Check sheet for the modelled part. Datum: model origin and axes. Units: mm. Coordinates: 2 decimals unless noted, no trailing zeros. Write each loop counter-clockwise with the first axis right and the second up, starting at its lowest first coordinate (ties: lowest second). Pieces come first, ordered by that corner, then holes. Notation, with made-up numbers: M 63.25,14.5 L 122.25,14.5 A9 ccw 122.25,20.5 Z; hole C 0,-29.75 d4. An arc over 180 degrees is marked long. Answer as CSV lines item,"result". Start each with the question number.
Q1. Sectioned sample at B-B, the plane x = 34. Record the cut outline in (y, z).
Q2. Thickness scan on line 1 along Y through (x, z) = (-60.5, -0.85); line 2 along Y through (x, z) = (-5, -0.9); line 3 along Y through (x, z) = (50, 0.05). Record the ranges inside material, lowest first. Write a range as from..to.
Q3. Sectioned sample at A-A, the plane x = 58.9. Record the cut outline in (y, z), then the cut area to 3 significant figures.
Q4. Sectioned sample at C-C, the plane y = 0.05. Record the cut outline in (x, z), then the cut area to 3 significant figures.
Q5. Sectioned sample at D-D, the plane z = -1.45. Count the separate pieces of the cut face and the enclosed holes in it, then the cut area to 3 significant figures.
Q6. Depth check by flat-ended pin: pin 1 Ø3.5 at (x, y) = (-45, 5) entering from +Z. Enter the tip coordinate at first touch or a pass-through.
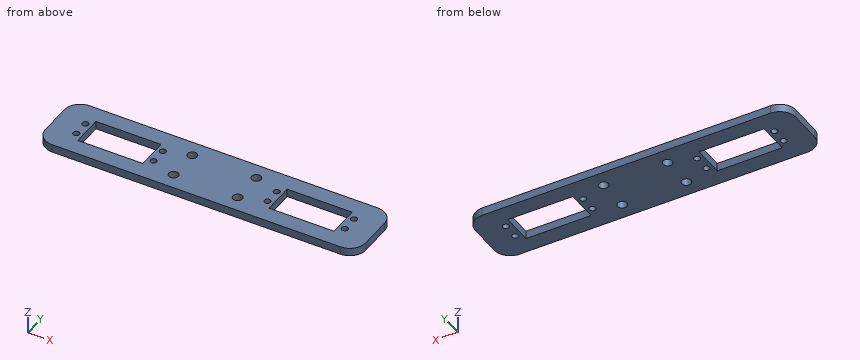
from build123d import *

# Parameters (mm, degrees)
CROQUIS1_W            = 200
CROQUIS1_H            = 40
EXTRUIR1_DEPTH        = 2.5
REDONDEO1_R           = 10
CROQUIS3_W            = 40.6
CROQUIS3_H            = 19.5
EXTRUIR2_DEPTH        = 10
CROQUIS4_R            = 1.95
CORTAR_EXTRUIR1_DEPTH = 10
CROQUIS5_R            = 2.95
CORTAR_EXTRUIR3_DEPTH = 10


with BuildPart() as part:
    # Croquis1 → Extruir1 (new, symmetric)
    with BuildSketch(Plane.XY):
        with Locations((-25, -5)):
            Rectangle(CROQUIS1_W, CROQUIS1_H)
    extrude(amount=EXTRUIR1_DEPTH, both=True)

    # Redondeo1
    redondeo1_edges = [part.edges().sort_by_distance(p)[0] for p in [
        (75, 15, 0),
        (75, -25, 0),
        (-125, -25, 0),
        (-125, 15, 0),
    ]]
    fillet(redondeo1_edges, radius=REDONDEO1_R)

    # Croquis3 → Extruir2 (cut)
    with BuildSketch(Plane.XY.offset(2.5)):
        with Locations((34.7, -5)):
            Rectangle(CROQUIS3_W, CROQUIS3_H)
        with Locations((-84.7, -5)):
            Rectangle(CROQUIS3_W, CROQUIS3_H)
    extrude(amount=-EXTRUIR2_DEPTH, mode=Mode.SUBTRACT)

    # Croquis4 → Cortar-Extruir1 (cut)
    with BuildSketch(Plane.XY.offset(2.5)):
        with Locations((58.9, -9.85)):
            Circle(CROQUIS4_R)
        with Locations((58.9, 0.05)):
            Circle(CROQUIS4_R)
        with Locations((10.6, 0.05)):
            Circle(CROQUIS4_R)
        with Locations((10.6, -9.85)):
            Circle(CROQUIS4_R)
        with Locations((-108.8, -9.85)):
            Circle(CROQUIS4_R)
        with Locations((-108.8, 0.05)):
            Circle(CROQUIS4_R)
        with Locations((-60.5, 0.05)):
            Circle(CROQUIS4_R)
        with Locations((-60.5, -9.85)):
            Circle(CROQUIS4_R)
    extrude(amount=-CORTAR_EXTRUIR1_DEPTH, mode=Mode.SUBTRACT)

    # Croquis5 → Cortar-Extruir3 (cut)
    with BuildSketch(Plane.XY.offset(2.5)):
        with Locations((-45, 5)):
            Circle(CROQUIS5_R)
        with Locations(Location((-45, -15, 0), (0, 0, 180))):
            Circle(CROQUIS5_R)
        with Locations((-5, -15)):
            Circle(CROQUIS5_R)
        with Locations(Location((-5, 5, 0), (0, 0, 180))):
            Circle(CROQUIS5_R)
    extrude(amount=-CORTAR_EXTRUIR3_DEPTH, mode=Mode.SUBTRACT)


solid = part.part
Output:
1,outline,"M -25,-2.5 L -14.75,-2.5 L -14.75,2.5 L -25,2.5 Z; M 4.75,-2.5 L 15,-2.5 L 15,2.5 L 4.75,2.5 Z"
2,line 1,"y = -25..-11.8, -7.9..-1.9, 2..15"
2,line 2,"y = -25..-17.95, -12.05..2.05, 7.95..15"
2,line 3,"y = -25..-14.75, 4.75..15"
3,outline,"M -25,-2.5 L -11.8,-2.5 L -11.8,2.5 L -25,2.5 Z; M -7.9,-2.5 L -1.9,-2.5 L -1.9,2.5 L -7.9,2.5 Z; M 2,-2.5 L 15,-2.5 L 15,2.5 L 2,2.5 Z"
3,area,"161 mm^2"
4,outline,"M -125,-2.5 L -110.75,-2.5 L -110.75,2.5 L -125,2.5 Z; M -106.85,-2.5 L -105,-2.5 L -105,2.5 L -106.85,2.5 Z; M -64.4,-2.5 L -62.45,-2.5 L -62.45,2.5 L -64.4,2.5 Z; M -58.55,-2.5 L 8.65,-2.5 L 8.65,2.5 L -58.55,2.5 Z; M 12.55,-2.5 L 14.4,-2.5 L 14.4,2.5 L 12.55,2.5 Z; M 55,-2.5 L 56.95,-2.5 L 56.95,2.5 L 55,2.5 Z; M 60.85,-2.5 L 75,-2.5 L 75,2.5 L 60.85,2.5 Z"
4,area,"516 mm^2"
5,separate pieces,"1"
5,enclosed holes,"14"
5,area,"6,130 mm^2"
6,pin 1,"passes through"
